from build123d import *

# Parameters (mm, degrees)
SKETCH1_R                            = 75.692
SKETCH1_R_2                          = 69.342
BOSS_EXTRUDE1_DEPTH                  = 22.225
SKETCH2_R                            = 75.692
BOSS_EXTRUDE2_DEPTH                  = 12.7
TAP_DRILL_FOR_1_4_20_TAP1_AT_2_COUNT = 2
TAP_DRILL_FOR_1_4_20_TAP1_AT_2_PITCH = 53.488399339
CIRPATTERN1_COUNT                    = 6
CUT_EXTRUDE1_DEPTH                   = 13.7000001
FILLET1_R                            = 1.5875
M4_CLEARANCE_HOLE1_D                 = 4.5
M4_CLEARANCE_HOLE1_DEPTH             = 12.7


with BuildPart() as part:
    # Sketch1 → Boss-Extrude1 (new body)
    with BuildSketch(Plane(origin=(0, 0, 0), x_dir=(1, 0, 0), z_dir=(0, 1, 0))):
        Circle(SKETCH1_R)
        Circle(SKETCH1_R_2, mode=Mode.SUBTRACT)
    extrude(amount=BOSS_EXTRUDE1_DEPTH)

    # Sketch2 → Boss-Extrude2 (add)
    with BuildSketch(Plane.XZ):
        Circle(SKETCH2_R)
    extrude(amount=BOSS_EXTRUDE2_DEPTH)

    # Sketch4 → Tap Drill for 1/4-20 Tap1 (revolve, cut)
    with BuildSketch(Plane(origin=(73.997176623, 4.896298223, 15.927859738), x_dir=(0.210429897, 0, -0.97760895), z_dir=(0, 1, 0))):
        Polygon((0, 0), (0, 11.185816902), (2.5527, 9.652), (2.5527, 0), align=None)
    tap_drill_for_1_4_20_tap1 = revolve(axis=Axis((80.204993454, 4.896298223, 17.264089582), (-0.97760895, 0, -0.210429897)), mode=Mode.SUBTRACT)

    # Tap Drill for 1/4-20 Tap1 at 2: Tap Drill for 1/4-20 Tap1 ×2
    with Locations(*[Vector(-0.110438581, 0.851210999, 0.51307227) * (i * TAP_DRILL_FOR_1_4_20_TAP1_AT_2_PITCH) for i in range(1, TAP_DRILL_FOR_1_4_20_TAP1_AT_2_COUNT)]):
        add(tap_drill_for_1_4_20_tap1, mode=Mode.SUBTRACT)

    # CirPattern1: Tap Drill for 1/4-20 Tap1 ×6 about axis
    cirpattern1_axis = Axis((0, 22.225, 0), (0, -1, 0))
    for i in range(1, CIRPATTERN1_COUNT):
        add(tap_drill_for_1_4_20_tap1.rotate(cirpattern1_axis, i * 360 / CIRPATTERN1_COUNT), mode=Mode.SUBTRACT)

    # CirPattern1 copy 1 sketch → CirPattern1 copy 1 (revolve, cut)
    with BuildSketch(Plane(origin=(-3.515628412, 50.426212075, 80.653301416), x_dir=(0.951849134, 0, -0.306566839), z_dir=(0, 1, 0))):
        Polygon((0, 0), (0, 11.185816902), (2.5527, 9.652), (2.5527, 0), align=None)
    revolve(axis=Axis((-1.568928987, 50.426212075, 86.697543415), (-0.306566839, 0, -0.951849134)), mode=Mode.SUBTRACT)

    # CirPattern1 copy 2 sketch → CirPattern1 copy 2 (revolve, cut)
    with BuildSketch(Plane(origin=(-71.605622131, 50.426212075, 37.282027193), x_dir=(0.741419237, 0, 0.671042111), z_dir=(0, 1, 0))):
        Polygon((0, 0), (0, 11.185816902), (2.5527, 9.652), (2.5527, 0), align=None)
    revolve(axis=Axis((-75.866739537, 50.426212075, 41.990039348), (0.671042111, 0, -0.741419237)), mode=Mode.SUBTRACT)

    # CirPattern1 copy 3 sketch → CirPattern1 copy 3 (revolve, cut)
    with BuildSketch(Plane(origin=(-68.089993719, 50.426212075, -43.371274223), x_dir=(-0.210429897, 0, 0.97760895), z_dir=(0, 1, 0))):
        Polygon((0, 0), (0, 11.185816902), (2.5527, 9.652), (2.5527, 0), align=None)
    revolve(axis=Axis((-74.29781055, 50.426212075, -44.707504067), (0.97760895, 0, 0.210429897)), mode=Mode.SUBTRACT)

    # CirPattern1 copy 4 sketch → CirPattern1 copy 4 (revolve, cut)
    with BuildSketch(Plane(origin=(3.515628412, 50.426212075, -80.653301416), x_dir=(-0.951849134, 0, 0.306566839), z_dir=(0, 1, 0))):
        Polygon((0, 0), (0, 11.185816902), (2.5527, 9.652), (2.5527, 0), align=None)
    revolve(axis=Axis((1.568928987, 50.426212075, -86.697543415), (0.306566839, 0, 0.951849134)), mode=Mode.SUBTRACT)

    # CirPattern1 copy 5 sketch → CirPattern1 copy 5 (revolve, cut)
    with BuildSketch(Plane(origin=(71.605622131, 50.426212075, -37.282027193), x_dir=(-0.741419237, 0, -0.671042111), z_dir=(0, 1, 0))):
        Polygon((0, 0), (0, 11.185816902), (2.5527, 9.652), (2.5527, 0), align=None)
    revolve(axis=Axis((75.866739537, 50.426212075, -41.990039348), (-0.671042111, 0, 0.741419237)), mode=Mode.SUBTRACT)

    # Sketch5 → Cut-Extrude1 (cut, through all)
    with BuildSketch(Plane(origin=(0, 0, 0), x_dir=(1, 0, 0), z_dir=(0, 1, 0))):
        Polygon((-52.650183893, -15.647551982), (-45.353610572, -9.525), (-12.7, -48.44005771), (-19.996573321, -54.562609693), align=None)
    extrude(amount=-CUT_EXTRUDE1_DEPTH, mode=Mode.SUBTRACT)

    # Fillet1
    fillet1_edges = [part.edges().sort_by_distance(p)[0] for p in [
        (-19.996573321, -6.35, 54.562609693),
        (-52.650183893, -6.35, 15.647551982),
        (-45.353610572, -6.35, 9.525),
        (-12.7, -6.35, 48.44005771),
    ]]
    fillet(fillet1_edges, radius=FILLET1_R)

    # M4 Clearance Hole1
    with Locations(Plane(origin=(0, 0, 0), x_dir=(1, 0, 0), z_dir=(0, 1, 0))):
        with Locations((-55.124449215, -5.28970267)):
            Hole(M4_CLEARANCE_HOLE1_D / 2, depth=M4_CLEARANCE_HOLE1_DEPTH)


solid = part.part
Part model, mm, in its own coordinate system. A direction names the side the tool comes from. Give positions to 0.01 mm unless a question says otherwise; leave off trailing zeros. Write each loop counter-clockwise with the first axis right and the second up, starting at its lowest first coordinate (ties: lowest second). Pieces come first, ordered by that corner, then holes.
1) Cut at C-C on x = 0. Write the cut outline in (y, z) (3 decimals).
Resolved:
outline: (-12.7, -75.692) - (22.225, -75.692) - (22.225, -69.342) - (0, -69.342) - (0, 69.342) - (22.225, 69.342) - (22.225, 75.692) - (-12.7, 75.692) - close
2) Two-plate mould, pull along Y, no slides. Class faces 4 (the face through (-1, 0, 1)), 5 (the face through (-36.11, -6.26, 35.36)), 6 (the face through (-71.203, 2.744, -13.923)): released by +Y, released by -Y, zero draft, split by the parting line, or undercut.
Resolved:
face 4: released by +Y
face 5: zero draft
face 6: undercut
3) Cut at B-B on z = 0. Write the cut outline in (x, y) (3 decimals), then the cut area to 3 significant figures.
Resolved:
outline: (-75.692, -12.7) - (75.692, -12.7) - (75.692, 22.225) - (69.342, 22.225) - (69.342, 0) - (-69.342, 0) - (-69.342, 22.225) - (-75.692, 22.225) - close
area: 2,200 mm2
4) Which spindle directions (+Z, -Z, +X, -X, +Y, -Y) get a long thin tool onto all of the face, cutting with end or side? Do faces 1 (the face through (-49.036, -6.261, 12.615)), 2 (the face through (-20.45, 3.17, -69.62)), 3 (the face through (-69.275, 10.957, -3.049)). Say none if no direction does.
Resolved:
face 1: +Y, -Y
face 2: none
face 3: +Y
5) Probe L1, parallel to Z at x = 0, y = 17; L2, parallel to Y at x = -27, z = 63. List the from-to ranges inside material, lowest first.
Resolved:
L1: z = -75.69 to -69.34, 69.34 to 75.69
L2: y = -12.7 to 0
6) Cut at A-A on x = -34.5. Write the cut outline in (y, z) (3 decimals), then the cut area to 3 significant figures.
Resolved:
outline: (-12.7, -67.372) - (22.225, -67.372) - (22.225, -60.15) - (0, -60.15) - (0, 22.46) - (-12.7, 22.46) - close; (-12.7, 37.278) - (0, 37.278) - (0, 60.15) - (22.225, 60.15) - (22.225, 67.372) - (-12.7, 67.372) - close
area: 1,840 mm2
7) Pin check, flat tips, straight feed: pin 1 (8 mm diameter, centred on y = 2, z = 47.5, fed in from +X); pin 2 (5 mm diameter, centred on y = -7, z = -21.5, fed in from +X); pin 3 (6 mm diameter, centred on x = -23, y = 10.5, fed in from +Z). Stop position of each tip, or through.
Resolved:
pin 1: stops at x = 61.94
pin 2: stops at x = 73.27
pin 3: stops at z = 73
8) Cut at D-D on y = 11. Write the cut outline in (x, z), then the cut area to 3 significant figures.
Resolved:
outline: circle Ø151.38 at (0, 0); hole circle Ø138.68 at (0, 0)
area: 2,890 mm2
